from build123d import *

# Parameters (mm, degrees)
PAD_DEPTH           = 43
HOLE_D              = 25
HOLE_CSINK_D        = 30
HOLE_CSINK_ANGLE    = 90
HOLE001_D           = 3.5
HOLE001_CBORE_D     = 5.5
HOLE001_CBORE_DEPTH = 15
SKETCH003_W         = 62.209956
SKETCH003_H         = 20.4
POCKET_DEPTH        = 5
POCKET_DEPTH_BACK   = 5
POCKET001_DEPTH     = 20
SKETCH005_W         = 20.4
SKETCH005_H         = 20.4
POCKET002_DEPTH     = 20
HOLE002_D           = 5.5
HOLE002_DEPTH       = 25
HOLE002_CBORE_D     = 9
HOLE002_CBORE_DEPTH = 15
CHAMFER_SIZE        = 1
SKETCH007_R         = 1.25
HOLE003_DEPTH       = 12
HOLE003_TIPS_R      = 1.25
POCKET003_DEPTH     = 2.5


with BuildPart() as part:
    # Sketch → Pad (new body)
    with BuildSketch(Plane.XY):
        Polygon((43, -20), (0, -20), (0, 0), (63, 0), (63, -50), (43, -50), align=None)
    extrude(amount=PAD_DEPTH)

    # Hole (through all)
    with Locations(Plane.XZ.offset(20)):
        with Locations((21.5, 21.5)):
            CounterSinkHole(HOLE_D / 2, HOLE_CSINK_D / 2, counter_sink_angle=HOLE_CSINK_ANGLE)

    # Hole001 (through all)
    with Locations(Plane.XZ.offset(20)):
        with Locations((6, 37), (37, 37), (37, 6), (6, 6)):
            CounterBoreHole(HOLE001_D / 2, HOLE001_CBORE_D / 2, HOLE001_CBORE_DEPTH)

    # Sketch003 (on Face1 of Hole001) → Pocket (cut, two sides)
    with BuildSketch(Plane.XZ.offset(20)) as pocket_sk:
        with Locations((54.005183, 21.5)):
            Rectangle(SKETCH003_W, SKETCH003_H)
    extrude(amount=-POCKET_DEPTH, mode=Mode.SUBTRACT)
    extrude(pocket_sk.sketch, amount=POCKET_DEPTH_BACK, mode=Mode.SUBTRACT)

    # Sketch004 (on Face3 of Pocket) → Pocket001 (cut)
    with BuildSketch(Plane(origin=(0, 0, 0), x_dir=(0, -1, 0), z_dir=(-1, 0, 0))):
        with BuildLine():
            ThreePointArc((14, 26.5), (9, 21.5), (14, 16.5))
            Line((20, 16.5), (14, 16.5))
            Line((20, 26.5), (20, 16.5))
            Line((14, 26.5), (20, 26.5))
        make_face()
    extrude(amount=-POCKET001_DEPTH, mode=Mode.SUBTRACT)

    # Sketch005 (on Face11 of Pocket001) → Pocket002 (cut)
    with BuildSketch(Plane.YZ.offset(63)):
        with Locations((-20, 21.5)):
            Rectangle(SKETCH005_W, SKETCH005_H)
    extrude(amount=-POCKET002_DEPTH, mode=Mode.SUBTRACT)

    # Hole002
    with Locations(Plane(origin=(43, 0, 0), x_dir=(0, -1, 0), z_dir=(-1, 0, 0))):
        with Locations((40.2, 21.5)):
            CounterBoreHole(HOLE002_D / 2, HOLE002_CBORE_D / 2, HOLE002_CBORE_DEPTH, depth=HOLE002_DEPTH)

    # Chamfer
    chamfer_edges = [part.edges().sort_by_distance(p)[0] for p in [
        (63, -27.6, 31.7),
        (63, -30.2, 21.5),
        (63, -20, 31.7),
        (63, -12.4, 31.7),
        (63, -9.8, 21.5),
        (63, -12.4, 11.3),
        (63, -20, 11.3),
        (63, -27.6, 11.3),
    ]]
    chamfer(chamfer_edges, length=CHAMFER_SIZE)

    # Sketch007 (on Face12 of Chamfer) → Hole003 (cut)
    with BuildSketch(Plane.XY.offset(43)):
        with Locations((55.7, -5.2)):
            Circle(SKETCH007_R)
        with Locations((55.7, -14.7)):
            Circle(SKETCH007_R)
    extrude(amount=-HOLE003_DEPTH, mode=Mode.SUBTRACT)

    # Hole003 tips → Hole003 tip 1 section 0
    with BuildSketch(Plane.XY.offset(31), mode=Mode.PRIVATE) as hole003_tip_1_s0:
        with Locations((55.7, -5.2)):
            Circle(HOLE003_TIPS_R)
    loft([hole003_tip_1_s0.sketch, Vertex(55.7, -5.2, 30.248924)], mode=Mode.SUBTRACT)

    # Hole003 tips → Hole003 tip 2 section 0
    with BuildSketch(Plane.XY.offset(31), mode=Mode.PRIVATE) as hole003_tip_2_s0:
        with Locations((55.7, -14.7)):
            Circle(HOLE003_TIPS_R)
    loft([hole003_tip_2_s0.sketch, Vertex(55.7, -14.7, 30.248924)], mode=Mode.SUBTRACT)

    # Sketch008 → Pocket003 (cut, symmetric)
    with BuildSketch(Plane.YZ.offset(21.5)):
        with BuildLine():
            ThreePointArc((-18, 35), (-13.757359, 36.757359), (-12, 41))
            Line((-12, 43), (-12, 41))
            Line((-12, 43), (-15, 43))
            Line((-15, 43), (-15, 41))
            ThreePointArc((-18, 38), (-15.87868, 38.87868), (-15, 41))
            Line((-18, 38), (-20, 38))
            Line((-20, 35), (-20, 38))
            Line((-18, 35), (-20, 35))
        make_face()
    extrude(amount=POCKET003_DEPTH, both=True, mode=Mode.SUBTRACT)


solid = part.part
Can you work these out from the model? Positions are in its coordinate system, mm. A direction names the side the tool comes from. Coordinates: 2 decimals unless noted, no trailing zeros. Loops run counter-clockwise (first coordinate to the right, second up) from the corner with the lowest first, then second, coordinate; pieces in that order, holes last. Notation, with made-up numbers: M -34,39 L 24,39 A20 ccw 24,52 Z; hole C 52.5,42.25 d2. An arc over 180 degrees is marked long. Return JSON: item names as keys, results as strings. Group by question number.
Item 1: Imagine slicing it at A-A (y = -40.2). Please give me the cut outline in (x, z), and give its area (4 significant figures).
Item 2: If I drill on L1, parallel to Z at x = 37, y = -2; L2, parallel to Z at x = 61, y = -40; L3, parallel to Z at x = 37, y = -16, over which ranges is the centre line in solid material (lowest first)? Write a range as from..to.
Item 3: On a 3-axis mill with a long thin cutter (end or side, diameter ignored), from which of +Z, -Z, +X, -X, +Y, -Y can I reach the whole of each face in a straight line? I mean faces 1 (the flat face through (53, -30.2, 21)), 2 (the cylindrical face through (5.642, -12.605, 39.727)), 3 (the flat face through (22, -20, 6)), 4 (the flat face through (43, -12, 22)). Say none if no direction works.
Item 4: Thinking about a two-plate mould opening in Z: for faces 5 (the flat face through (17, -20, 36)), 6 (the flat face through (58, -42, 24)), which applies, released by +Z, released by -Z, zero draft, split by the parting line, or undercut?
Item 5: Imagine slicing it at C-C (x = 51.5). Please give me the cut outline in (y, z), and give its area (3 significant figures).
Item 6: Imagine slicing it at D-D (y = -11). Please give me the cut outline in (x, z).
Item 7: Imagine slicing it at B-B (x = 37). Please give me the cut outline in (y, z), and give its area (3 significant figures).
Item 8: I'm going to push flat-ended pins straight in: pin 1 Ø2 at (x, z) = (39, 32) entering from -Y; pin 2 Ø2.5 at (y, z) = (-38.5, 23.5) entering from -X; pin 3 Ø4 at (y, z) = (-35, 27) entering from -X. Where does each tip first touch, or does it pass through?
Verdict:
{
 "1": {"outline": "M 43,0 L 63,0 L 63,18.75 L 58,18.75 L 58,17 L 43,17 Z; M 43,26 L 58,26 L 58,24.25 L 63,24.25 L 63,43 L 43,43 Z", "area": "697.5 mm^2"},
 "2": {"L1": "z = 0..4.25, 7.75..35.25, 38.75..43", "L2": "z = 0..18.76, 24.24..43", "L3": "z = 0..3.25, 8.75..11.3, 31.7..34.25, 39.75..43"},
 "3": {"face 1": "+X, -X", "face 2": "-Y", "face 3": "+Z, -Z, -X, -Y", "face 4": "+X"},
 "4": {"face 5": "zero draft", "face 6": "undercut"},
 "5": {"outline": "M -50,0 L 0,0 L 0,43 L -50,43 Z; hole C -40.2,21.5 d9; hole M -30.2,11.3 L -9.8,11.3 L -9.8,31.7 L -30.2,31.7 Z", "area": "1,670 mm^2"},
 "6": {"outline": "M 0,0 L 63,0 L 63,10.3 L 62,11.3 L 43,11.3 L 43,31.7 L 62,31.7 L 63,32.7 L 63,43 L 0,43 L 0,25.5 L 9.66,25.5 A12.5 cw long 9.66,17.5 L 0,17.5 Z; hole C 6,6 d5.5; hole C 6,37 d5.5; hole C 37,6 d5.5; hole C 37,37 d5.5"},
 "7": {"outline": "M -20,0 L 0,0 L 0,4.25 L -5,4.25 L -5,3.25 L -20,3.25 Z; M -20,8.75 L -5,8.75 L -5,7.75 L 0,7.75 L 0,35.25 L -5,35.25 L -5,34.25 L -20,34.25 L -20,31.7 L -15,31.7 L -15,11.3 L -20,11.3 Z; M -20,39.75 L -5,39.75 L -5,38.75 L 0,38.75 L 0,43 L -20,43 Z", "area": "558 mm^2"},
 "8": {"pin 1": "stops at y = -20", "pin 2": "stops at x = 58", "pin 3": "stops at x = 43"}
}
